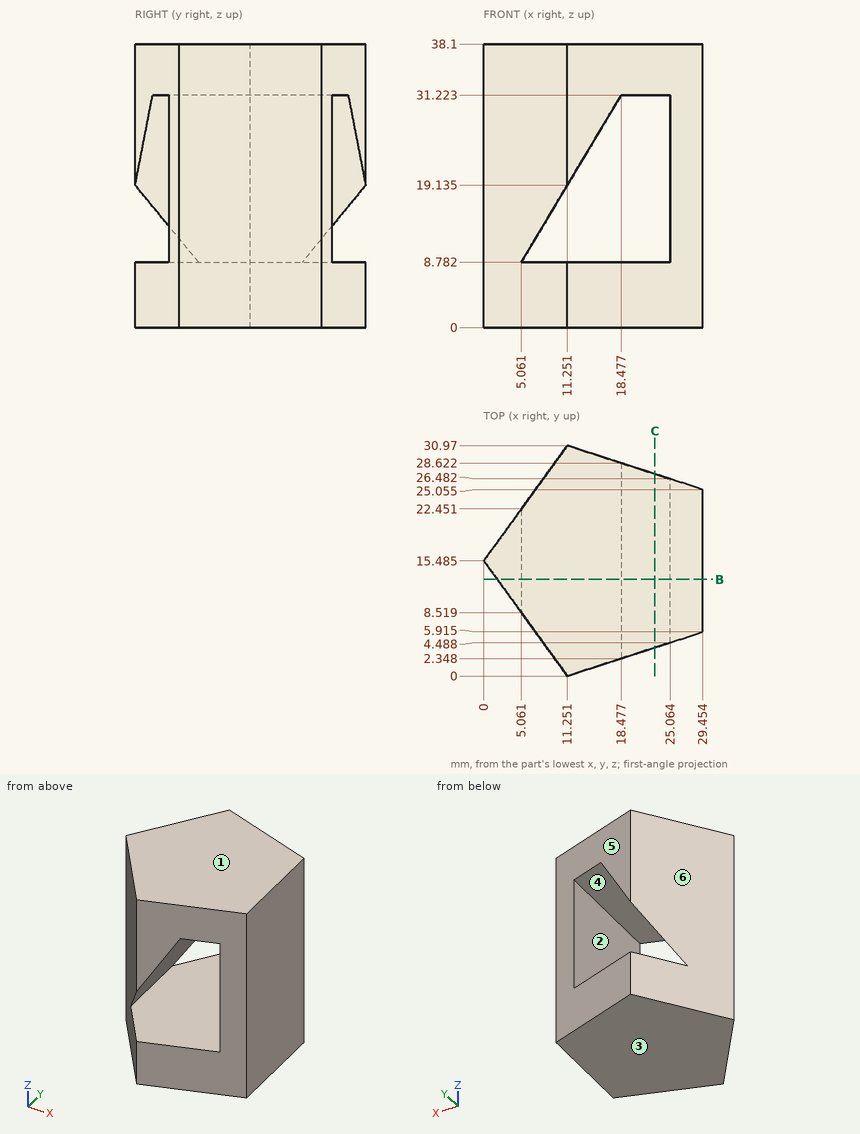
Can you work these out from the drawing? Everything is in mm from the part's minimum corner. A direction names the side the tool comes from. Round coordinates to 2 decimals unless told otherwise and drop trailing zeros. Write each loop counter-clockwise with the first axis right and the second up, starting at its lowest first coordinate (ties: lowest second). Pieces come first, ordered by that corner, then holes. Notation, with made-up numbers: (-31, -36.75) - (-20, -36.75) arc R20 ccw to (-20, -18.75) - close; hole circle Ø2 at (34, 60). An arc over 180 degrees is marked (long way). Write each question's results on one line, items separated by ' | '. Start each with the question number.
1) We'd pull the mould along X, two halves only. Please class the marked faces 3, 4, 5 and 6: released by +X, released by -X, zero draft, split by the parting line, or undercut.
2) Please list where these lines run through material, in increasing order: line 1 (Z direction, x = 19.5, y = 5.5); line 2 (X direction, y = 11, z = 18.5) (1 decimal); line 3 (Z direction, x = 12, y = 15) (1 decimal).
3) For pin 1 Ø2 at (x, z) = (13, 29) entering from -Y; pin 2 Ø4 at (x, z) = (26, 6) entering from +Y; pin 3 Ø11 at (y, z) = (19, 18.5) entering from -X, each with a flat end and sliding along its axis, tell me the tip position at first contact or that it passes through.
4) Suppose I cut it at C-C (x = 23). List the corners of the cut face in (y, z) for me.
5) Which directions (+Z, -Z, +X, -X, +Y, -Y) give clear straight access to the entire face, cutting with the end or side of a thin tool? Please do the marked faces 1 and 2.
6) Suppose I cut it at B-B (y = 13). List the corners of the cut face in (x, z) for me (1 decimal), and give its area (3 significant figures).
Here are the results:
1) face 3: zero draft | face 4: undercut | face 5: released by +X | face 6: released by -X
2) line 1: z = 0 to 8.78, 31.22 to 38.1 | line 2: x = 3.3 to 10.9, 25.1 to 29.5 | line 3: z = 0 to 8.8, 20.4 to 38.1
3) pin 1: stops at y = 0.24 | pin 2: stops at y = 26.83 | pin 3: stops at x = 0
4) outline: (3.82, 0) - (27.15, 0) - (27.15, 8.78) - (3.82, 8.78) - close; (3.82, 31.22) - (27.15, 31.22) - (27.15, 38.1) - (3.82, 38.1) - close
5) face 1: +Z, +X, -X, +Y, -Y | face 2: +Y, -Y
6) outline: (1.8, 0) - (29.5, 0) - (29.5, 38.1) - (1.8, 38.1) - close; hole (5.1, 8.8) - (25.1, 8.8) - (25.1, 31.2) - (18.5, 31.2) - close | area: 755 mm2
